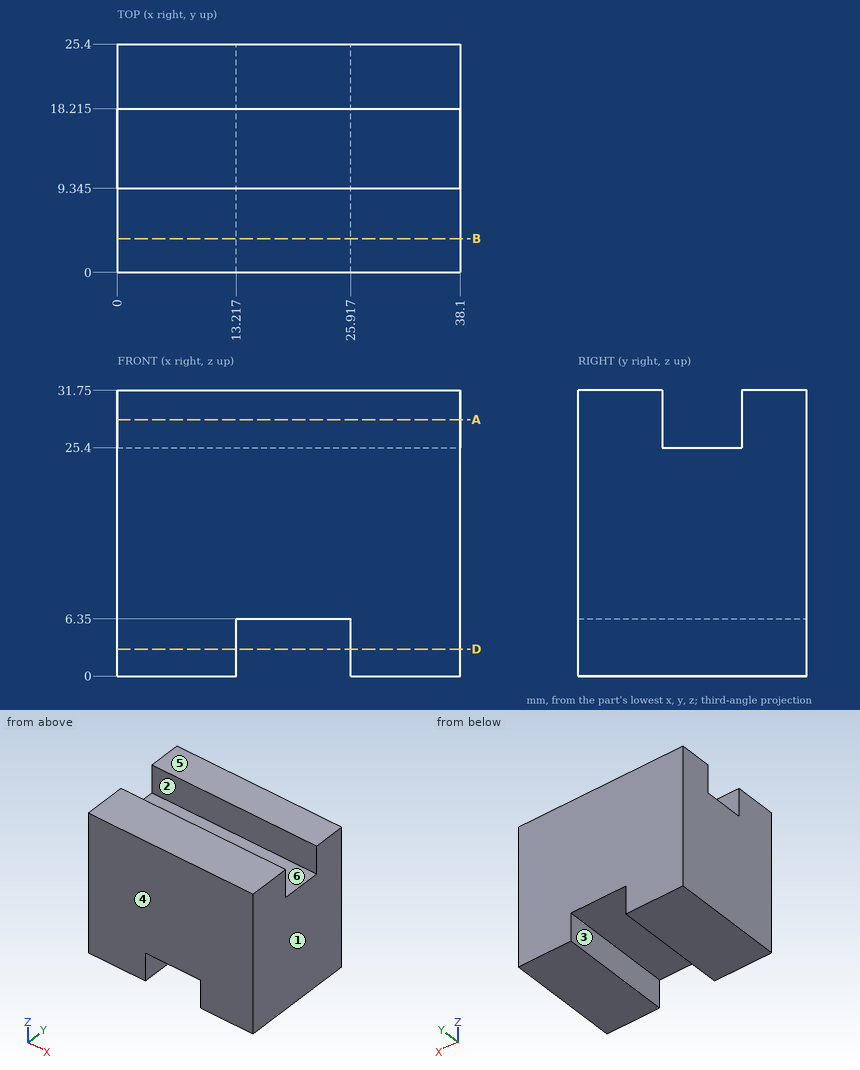
Here's the drawing with two shaded views (mm, measured from the low corner). I have some questions. A direction names the side the tool comes from. Give positions to 0.01 mm unless a question says otherwise; leave off trailing zeros. Write each loop counter-clockwise with the first axis right and the second up, starting at its lowest first coordinate (ties: lowest second). Pieces come first, ordered by that corner, then holes. Notation, with made-up numbers: (42, 72.5) -> (49, 72.5) arc R18 cw to (49, 107.5) -> close; hole circle Ø10 at (63.5, -4.5). An arc over 180 degrees is marked (long way). Use one line per item in the form item = value. Start each with the question number.
1. If I drill on L1, parallel to Y at x = 5.5, z = 30 (1 decimal); L2, parallel to X at y = 2.75, z = 3; L3, parallel to Z at x = 18, y = 12, over which ranges is the centre line in solid material (lowest first)?
2. Imagine slicing it at D-D on z = 3. List the corners of the cut face in (x, y) for me.
3. On a 3-axis mill with a long thin cutter (end or side, diameter ignored), from which of +Z, -Z, +X, -X, +Y, -Y can I reach the whole of each face in a straight line? I mean the marked faces 1, 2 and 3. Say none if no direction works.
4. Imagine slicing it at B-B on y = 3.75. List the corners of the cut face in (x, z) for me.
5. Will this pin go through, and if not, where does the flat tip stop? pin 1 Ø6.5 at (x, y) = (17.5, 13.5) entering from -Z.
6. Imagine slicing it at A-A on z = 28.5. List the corners of the cut face in (x, y) for me (1 decimal).
7. Thinking about a two-plate mould opening in Y: for the marked faces 4, 5 and 6, which applies, +Y half, -Y half, draft (parallel to the pull), parting line (faces both ways), or undercut?
Entries:
q1.L1 = 0 to 9.3, 18.2 to 25.4
q1.L2 = 0 to 13.22, 25.92 to 38.1
q1.L3 = 6.35 to 25.4
q2.outline = (0, 0) -> (13.22, 0) -> (13.22, 25.4) -> (0, 25.4) -> close; (25.92, 0) -> (38.1, 0) -> (38.1, 25.4) -> (25.92, 25.4) -> close
q3.face_1 = +Z, -Z, +X, +Y, -Y
q3.face_2 = +Z, +X, -X
q3.face_3 = -Z, +Y, -Y
q4.outline = (0, 0) -> (13.22, 0) -> (13.22, 6.35) -> (25.92, 6.35) -> (25.92, 0) -> (38.1, 0) -> (38.1, 31.75) -> (0, 31.75) -> close
q5.pin_1 = 6.35
q6.outline = (0, 0) -> (38.1, 0) -> (38.1, 9.3) -> (0, 9.3) -> close; (0, 18.2) -> (38.1, 18.2) -> (38.1, 25.4) -> (0, 25.4) -> close
q7.face_4 = -Y half
q7.face_5 = draft
q7.face_6 = undercut
